Can you work these out from the model? Positions are in its coordinate system, mm. Face numbers are marked on the shaded views. Round coordinates to 2 decimals unless told otherwise and drop trailing zeros. Loops run counter-clockwise (first coordinate to the right, second up) from the corner with the lowest first, then second, coordinate; pieces in that order, holes last.
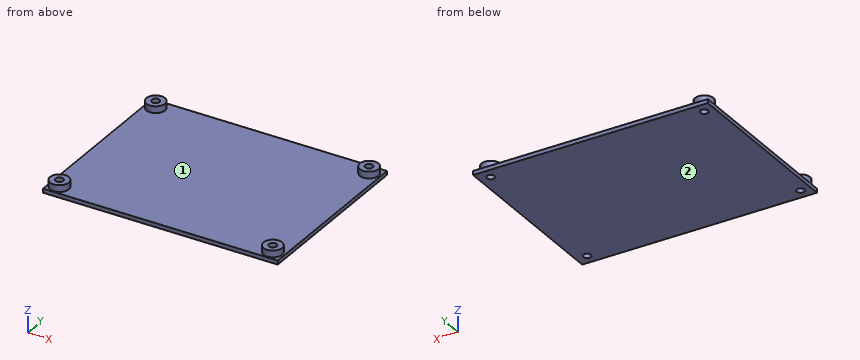
from build123d import *

# Parameters (mm, degrees)
F0_W     = 88
F0_H     = 67
F1_DEPTH = 1.5
F2_R     = 3.5
F3_DEPTH = 4
F4_R     = 1.45
F5_R     = 1.45
F6_R     = 1.45
F7_R     = 1.45
F8_DEPTH = 5


with BuildPart() as f1:
    # F0 (on Top) → F1 (new body)
    with BuildSketch(Plane.XY):
        with Locations((0, -0.916107)):
            Rectangle(F0_W, F0_H)
    extrude(amount=F1_DEPTH)

    # F2 (on face) → F3 (join)
    with BuildSketch(Plane.XY):
        with Locations((-40.190587, 28.489581)):
            Circle(F2_R)
        with Locations((39.809413, 28.488207)):
            Circle(F2_R)
        with Locations((-40.23079, -30.510419)):
            Circle(F2_R)
        with Locations((39.76921, -30.511793)):
            Circle(F2_R)
    extrude(amount=F3_DEPTH)

    # F4 (on face) + F5 (on face) + F6 (on face) + F7 (on face) → F8 (cut)
    with BuildSketch(Plane.XY.offset(4)):
        with Locations((-40.23079, -30.510419)):
            Circle(F4_R)
    with BuildSketch(Plane.XY.offset(4)):
        with Locations((-40.190587, 28.489581)):
            Circle(F5_R)
    with BuildSketch(Plane.XY.offset(4)):
        with Locations((39.76921, -30.511793)):
            Circle(F6_R)
    with BuildSketch(Plane.XY.offset(4)):
        with Locations((39.809413, 28.488207)):
            Circle(F7_R)
    extrude(amount=-F8_DEPTH, mode=Mode.SUBTRACT)


solid = f1.part
(1) If we section it at A-A, the plane z = 2.85: List the corners of the cut face in (x, y) for me.
Worked answers:
outline: circle Ø7 at (-40.23, -30.51); circle Ø7 at (-40.19, 28.49); circle Ø7 at (39.77, -30.51); circle Ø7 at (39.81, 28.49); hole circle Ø2.9 at (-40.23, -30.51); hole circle Ø2.9 at (-40.19, 28.49); hole circle Ø2.9 at (39.77, -30.51); hole circle Ø2.9 at (39.81, 28.49)
(2) If we mould it in two halves opening along X, with no side actions, what happens to the marked faces 1 and 2? For each: released by +X, released by -X, zero draft, split by the parting line, or undercut.
Worked answers:
face 1: undercut
face 2: zero draft
(3) Will these pins go through, and if not, where does the flat tip stop? P1, Ø1.7, axis at x = 39.81, y = 28.49, coming from the +Z side (3 decimals); P2, Ø12, axis at x = 22, y = 19.5, coming from the +Z side; P3, Ø4.5, axis at x = -40.23, y = -30.51, coming from the -Z side.
Worked answers:
P1: passes through
P2: stops at z = 1.5
P3: stops at z = 0
(4) If we section it at B-B, the plane y = -21: List the corners of the cut face in (x, z) for me.
Worked answers:
outline: (-44, 0) - (44, 0) - (44, 1.5) - (-44, 1.5) - close
(5) If we section it at C-C, the plane x = 24: List the corners of the cut face in (y, z) for me, then the cut area to 4 significant figures.
Worked answers:
outline: (-34.42, 0) - (32.58, 0) - (32.58, 1.5) - (-34.42, 1.5) - close
area: 100.5 mm2
(6) If I drill on line 1 (Z direction, x = 34.5, y = -26.5); line 2 (Y direction, x = -39, z = 2.5); line 3 (X direction, y = -30, z = 1.3), over which ranges is the centre line in solid material (lowest first)?
Worked answers:
line 1: z = 0 to 1.5
line 2: y = -33.79 to -31.28, -29.74 to -27.23, 25.2 to 27.66, 29.32 to 31.78
line 3: x = -44 to -41.59, -38.87 to 38.41, 41.13 to 44
